Part model, mm, in its own coordinate system. A direction names the side the tool comes from. Round coordinates to 2 decimals unless told otherwise and drop trailing zeros. Write each loop counter-clockwise with the first axis right and the second up, starting at its lowest first coordinate (ties: lowest second). Pieces come first, ordered by that corner, then holes.
```python
from build123d import *

# Parameters (mm, degrees)
FILLET_2_R               = 2
CHAMFER_2_SIZE           = 1
SKETCH_1_8_W             = 12
SKETCH_1_8_H             = 10
PATTERN_CIRCULAR_1_COUNT = 6
CUT_EXTRUDE_1_DEPTH      = 109.972473589


with BuildPart() as part:
    # Sketch 1 → Revolve 1 (revolve)
    with BuildSketch(Plane.XY, mode=Mode.PRIVATE) as revolve_1_sk:
        Polygon((0, 25), (50, 25), (50, 40), (12, 40), (12, 75), (0, 75), align=None)
    revolve(revolve_1_sk.sketch.rotate(Axis((0, 0, 0), (1, 0, 0)), 90), axis=Axis((0, 0, 0), (1, 0, 0)))

    # Fillet 2
    fillet_2_edges = [part.edges().sort_by_distance(p)[0] for p in [
        (12, 0, -40),
    ]]
    fillet(fillet_2_edges, radius=FILLET_2_R)

    # Chamfer 2
    chamfer_2_edges = [part.edges().sort_by_distance(p)[0] for p in [
        (0, 0, -75),
        (12, 0, -75),
        (50, 0, -40),
    ]]
    chamfer(chamfer_2_edges, length=CHAMFER_2_SIZE)

    # Sketch 1_8 → Cut-Revolve 1 (revolve, cut)
    with BuildSketch(Plane.XY, mode=Mode.PRIVATE) as cut_revolve_1_sk:
        with Locations((6, 60)):
            Rectangle(SKETCH_1_8_W, SKETCH_1_8_H)
    cut_revolve_1 = revolve(cut_revolve_1_sk.sketch.rotate(Axis((-8.265772118, 55, 0), (1, 0, 0)), 90), axis=Axis((-8.265772118, 55, 0), (1, 0, 0)), mode=Mode.SUBTRACT)

    # Pattern Circular 1: Cut-Revolve 1 ×6 about axis
    pattern_circular_1_axis = Axis((0, 0, 0), (1, 0, 0))
    for i in range(1, PATTERN_CIRCULAR_1_COUNT):
        add(cut_revolve_1.rotate(pattern_circular_1_axis, i * 360 / PATTERN_CIRCULAR_1_COUNT), mode=Mode.SUBTRACT)

    # Sketch 2 → Cut-Revolve 3 (revolve, cut)
    with BuildSketch(Plane(origin=(0, 0, 0), x_dir=(1, 0, 0), z_dir=(0, 1, 0))):
        Polygon((47, 25), (50, 25), (50, 30.196152423), align=None)
    revolve(axis=Axis((0, 0, 0), (1, 0, 0)), mode=Mode.SUBTRACT)

    # Sketch 3 → Cut-Extrude 1 (cut, through all)
    with BuildSketch(Plane(origin=(25, 0, 0), x_dir=(0, 0, -1), z_dir=(1, 0, 0))):
        Polygon((0, 35), (-30.310889132, 17.5), (-30.310889132, -17.5), (0, -35), (30.310889132, -17.5), (30.310889132, 17.5), align=None)
    extrude(amount=-CUT_EXTRUDE_1_DEPTH, mode=Mode.SUBTRACT)


solid = part.part
```
Q1. Cut at C-C on y = -27.5. State how many separate pieces and enclosed holes the cut face has, plus the area to 3 significant figures.
Values follow:
separate pieces: 3
enclosed holes: 0
area: 2,730 mm2
Q2. Drop flat-ended pins along their axis: pin 1 (18 mm diameter, centred on y = 5.5, z = -10, fed in from -X); pin 2 (3 mm diameter, centred on x = 28, z = -17.5, fed in from +Y); pin 3 (1 mm diameter, centred on x = 7, z = 30, fed in from +Y); pin 4 (3 mm diameter, centred on x = 34.5, y = -27.5, fed in from -Z). Give the stop position or say it passes through.
Values follow:
pin 1: passes through
pin 2: stops at y = 36.66
pin 3: stops at y = 68.95
pin 4: stops at z = -30.4
Q3. Cut at A-A on x = 23. Write the cut outline in (y, z).
Values follow:
outline: circle Ø80 at (0, 0); hole (-35, 0) - (-17.5, -30.31) - (17.5, -30.31) - (35, 0) - (17.5, 30.31) - (-17.5, 30.31) - close
Q4. Wall check: L1, parallel to Y at x = 7, z = 8; L2, parallel to X at y = -8.5, z = -41; L3, parallel to Z at x = 7.5, y = 20. Give the ranges that are in metal, low to high.
Values follow:
L1: y = -74.57 to -61, -49 to -30.38, 30.38 to 49, 61 to 74.57
L2: x = 0 to 12
L3: z = -72.28 to -54.25, -41.02 to -25.98, 25.98 to 41.02, 54.25 to 72.28
Q5. Which spindle directions (+Z, -Z, +X, -X, +Y, -Y) get a long thin tool onto all of the face, cutting with end or side? Do faces 1 (the flat face through (12, 32, -32)), 2 (the cylindrical face through (6.084, 23.67, 38.394)), 3 (the flat face through (12.675, 26.372, 14.943)). Say none if no direction does.
Values follow:
face 1: +X
face 2: +X, -X
face 3: -X
Q6. Cut at B-B on y = 0. Write the cut outline in (x, z).
Values follow:
outline: (0, -74) - (1, -75) - (11, -75) - (12, -74) - (12, -42) arc R2 cw to (14, -40) - (49, -40) - (50, -39) - (50, -30.2) - (47, -25) - (25, -25) - (25, -30.31) - (0, -30.31) - close; (0, 30.31) - (25, 30.31) - (25, 25) - (47, 25) - (50, 30.2) - (50, 39) - (49, 40) - (14, 40) arc R2 cw to (12, 42) - (12, 74) - (11, 75) - (1, 75) - (0, 74) - close
Q7. Cut at D-D on x = 39. Write the cut outline in (y, z).
Values follow:
outline: circle Ø80 at (0, 0); hole circle Ø50 at (0, 0)
Q8. Mould opens along Y. For faces 4 (the cylindrical face through (5.93, 66.538, 34.608)), 5 (the flat face through (50, 23, -20)), 6 (the cylindrical face through (6.08, -35.93, 53.01)) say: +Y half, -Y half, draft (parallel to the pull), parting line (faces both ways), or undercut.
Values follow:
face 4: parting line
face 5: draft
face 6: undercut
